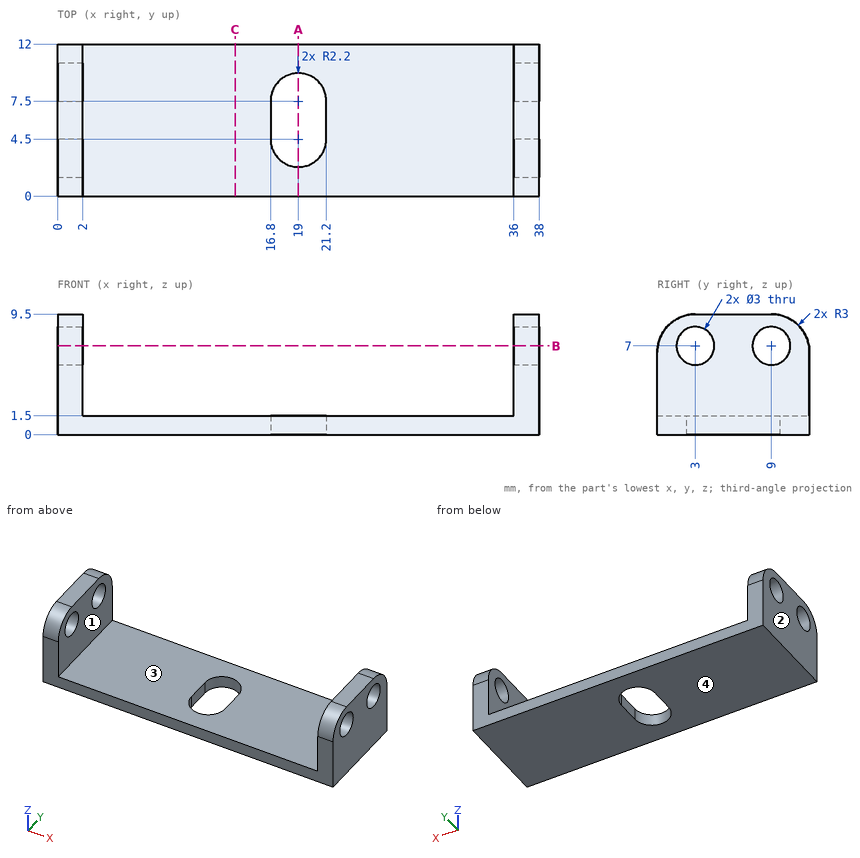
Can you work these out from the drawing? Everything is in mm from the part's minimum corner. Coordinates: 2 decimals unless noted, no trailing zeros. Write each loop counter-clockwise with the first axis right and the second up, starting at its lowest first coordinate (ties: lowest second). Pieces come first, ordered by that corner, then holes. Notation, with made-up numbers: (26.5, -17.5) - (64.5, -17.5) arc R7 ccw to (64.5, -4.5) - close; hole circle Ø10 at (47, 77). An arc over 180 degrees is marked (long way). One line per item, written item: value.
1) I need wall thicknesses on line 1 along X through (y, z) = (6, 5.5); line 2 along Y through (x, z) = (19, 1.25); line 3 along Z through (x, y) = (36.6, 9). Which ranges of each line are inside material? Lowest first, please.
Model answer:
line 1: x = 0 to 2, 36 to 38
line 2: y = 0 to 2.3, 9.7 to 12
line 3: z = 0 to 5.5, 8.5 to 9.5
2) I'm going to push flat-ended pins straight in: P1, Ø4, axis at y = 6.5, z = 3.5, coming from the -X side; P2, Ø1, axis at x = 19.5, y = 5, coming from the +Z side; P3, Ø1, axis at x = 21.5, y = 8.5, coming from the +Z side. Where does each tip first touch, or does it pass through?
Model answer:
P1: stops at x = 0
P2: passes through
P3: stops at z = 1.5
3) We'd pull the mould along X, two halves only. Please class the marked faces 1, 2, 3 and 4: pulls with the +X half, pulls with the -X half, needs draft (parallel to the pull), parting line crosses it, or undercut.
Model answer:
face 1: undercut
face 2: pulls with the -X half
face 3: undercut
face 4: needs draft
4) Suppose I cut it at C-C on x = 14. Write out the boundary of the cut face in (y, z).
Model answer:
outline: (0, 0) - (12, 0) - (12, 1.5) - (0, 1.5) - close
5) Suppose I cut it at A-A on x = 19. Write out the boundary of the cut face in (y, z), and give its area (3 significant figures).
Model answer:
outline: (0, 0) - (2.3, 0) - (2.3, 1.5) - (0, 1.5) - close; (9.7, 0) - (12, 0) - (12, 1.5) - (9.7, 1.5) - close
area: 6.90 mm²
6) Suppose I cut it at B-B on z = 7. Write out the boundary of the cut face in (x, y).
Model answer:
outline: (0, 0.04) - (2, 0.04) - (2, 1.5) - (0, 1.5) - close; (0, 4.5) - (2, 4.5) - (2, 7.5) - (0, 7.5) - close; (0, 10.5) - (2, 10.5) - (2, 11.96) - (0, 11.96) - close; (36, 0.04) - (38, 0.04) - (38, 1.5) - (36, 1.5) - close; (36, 4.5) - (38, 4.5) - (38, 7.5) - (36, 7.5) - close; (36, 10.5) - (38, 10.5) - (38, 11.96) - (36, 11.96) - close
